Design review of the part shown in the three views and the two pictorial views. Dimensions are in mm from the part's minimum x, y and z. A direction names the side the tool comes from. Round coordinates to 2 decimals unless told otherwise and drop trailing zeros. Order: outer loops, then holes, each group sorted by start corner. A loop starts at its lowest first (then second) coordinate and runs counter-clockwise, first axis right, second up. Notation, with made-up numbers: (38.5, 76) -> (45.5, 76) arc R18 ccw to (45.5, 99) -> close; hole circle Ø11 at (25.5, 41). An arc over 180 degrees is marked (long way). Put each result on its own line as item: value. Start each with the question number.
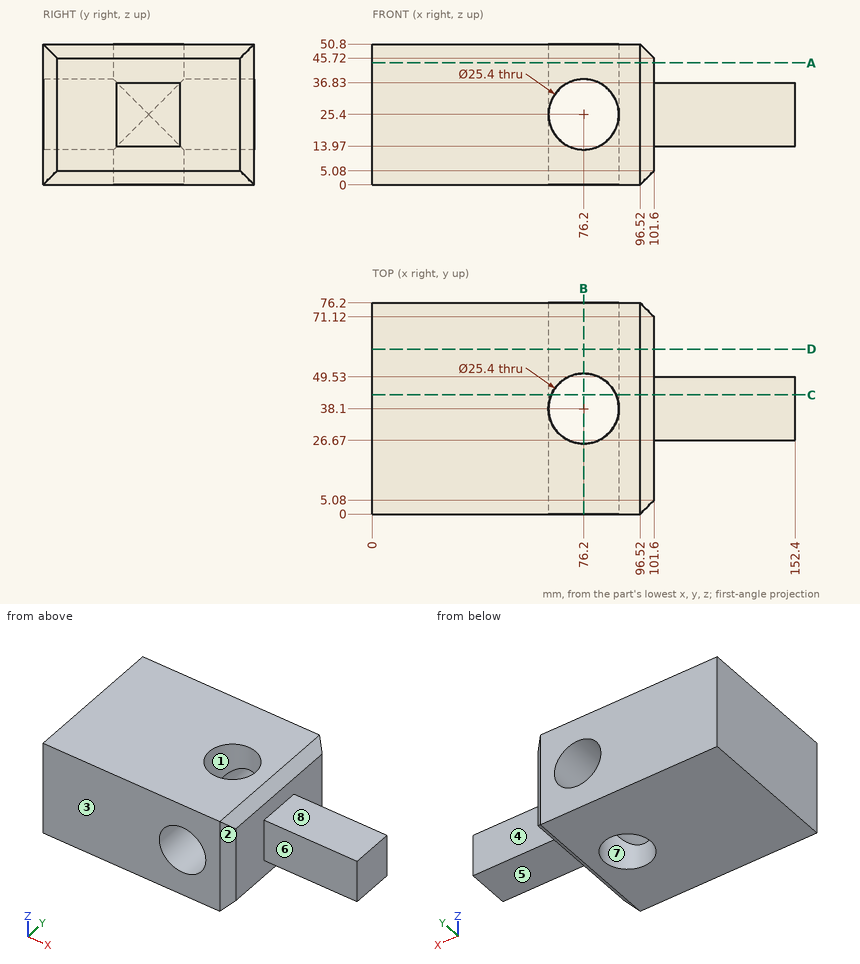
Q1. Take a section at C-C on y = 43. Give the boundary of the cut face in (x, z).
Q2. Wall thickness on probe 1 along X at (y, z) = (19, 25); probe 2 along Z at (x, y) = (76.2, 60); probe 3 along Y at (x, z) = (76.2, 40.5): over which ranges is each line inside the solid? List them lowest first. Write a range as [from, to].
Q3. For the marked faces 4, 5, 6, 7 and 8, list the 3-axis set-ups (+Z, -Z, +X, -X, +Y, -Y) from which the entire face can be reached by the end or side of a thin tool; tool diameter is ignored.
Q4. Clearance check with flat-ended pins moving along their axes: pin 1 Ø11.5 at (x, z) = (122.5, 24) entering from -Y; pin 2 Ø8 at (x, z) = (113.5, 22.5) entering from +Y; pin 3 Ø2 at (x, z) = (98, 27) entering from -Y. State where each tip first meets the part, or that it passes through.
Q5. Take a section at B-B on x = 76.2. Give the boundary of the cut face in (y, z).
Q6. Draft analysis for pull direction X (two halves, no side actions). For the marked faces 1, 2 and 3, state which applies: +X half, -X half, draft (parallel to the pull), parting line (faces both ways), or undercut.
Q7. Take a section at D-D on y = 59.5. Give the boundary of the cut face in (x, z).
Q8. Take a section at A-A on z = 44. Give the boundary of the cut face in (x, y), and give its area (3 significant figures).
Calculated:
1. outline: (0, 0) -> (64.48, 0) -> (64.48, 20.5) arc R12.7 cw to (64.48, 30.3) -> (64.48, 50.8) -> (0, 50.8) -> close; (87.92, 0) -> (96.52, 0) -> (101.6, 5.08) -> (101.6, 13.97) -> (152.4, 13.97) -> (152.4, 36.83) -> (101.6, 36.83) -> (101.6, 45.72) -> (96.52, 50.8) -> (87.92, 50.8) -> (87.92, 30.3) arc R12.7 cw to (87.92, 20.5) -> close
2. probe 1: x = [0, 63.51], [88.89, 101.6]
2. probe 2: z = [0, 12.7], [38.1, 50.8]
2. probe 3: y = [0, 25.4], [50.8, 76.2]
3. face 4: +Z, -Z, +X, +Y
3. face 5: -Z, +X, +Y, -Y
3. face 6: +Z, -Z, +X, -Y
3. face 7: +Z, -Z
3. face 8: +Z, +X, +Y, -Y
4. pin 1: stops at y = 26.67
4. pin 2: stops at y = 49.53
4. pin 3: stops at y = 0.48
5. outline: (0, 0) -> (25.4, 0) -> (25.4, 12.7) -> (0, 12.7) -> close; (0, 38.1) -> (25.4, 38.1) -> (25.4, 50.8) -> (0, 50.8) -> close; (50.8, 0) -> (76.2, 0) -> (76.2, 12.7) -> (50.8, 12.7) -> close; (50.8, 38.1) -> (76.2, 38.1) -> (76.2, 50.8) -> (50.8, 50.8) -> close
6. face 1: undercut
6. face 2: +X half
6. face 3: draft
7. outline: (0, 0) -> (96.52, 0) -> (101.6, 5.08) -> (101.6, 45.72) -> (96.52, 50.8) -> (0, 50.8) -> close; hole circle Ø25.4 at (76.2, 25.4)
8. outline: (0, 0) -> (96.52, 0) -> (101.6, 5.08) -> (101.6, 71.12) -> (96.52, 76.2) -> (0, 76.2) -> close; hole circle Ø25.4 at (76.2, 38.1)
8. area: 7,210 mm²
